```python
from build123d import *

# Parameters (mm, degrees)
SKETCH1_W           = 110
SKETCH1_H           = 150
BOSS_EXTRUDE1_DEPTH = 10
SKETCH2_W           = 9.95
SKETCH2_H           = 11
BOSS_EXTRUDE2_DEPTH = 7
SKETCH3_W           = 19.95
SKETCH3_H           = 11
SKETCH3_W_2         = 20
BOSS_EXTRUDE3_DEPTH = 6.95
SKETCH6_R           = 1.425
CUT_EXTRUDE1_DEPTH  = 10
SKETCH7_W           = 110
SKETCH7_H           = 1
BOSS_EXTRUDE4_DEPTH = 2


with BuildPart() as part:
    # Sketch1 → Boss-Extrude1 (new body)
    with BuildSketch(Plane.XY):
        with Locations((-38.267930395, -69.615981522)):
            Rectangle(SKETCH1_W, SKETCH1_H)
    extrude(amount=BOSS_EXTRUDE1_DEPTH)

    # Sketch2 → Boss-Extrude2 (add)
    with BuildSketch(Plane.XY.offset(10)):
        with Locations((-63.252930395, -0.115981522)):
            Rectangle(SKETCH2_W, SKETCH2_H)
        with Locations((-13.302930395, -0.115981522)):
            Rectangle(SKETCH2_W, SKETCH2_H)
    boss_extrude2 = extrude(amount=BOSS_EXTRUDE2_DEPTH)

    # Sketch3 → Boss-Extrude3 (add)
    with BuildSketch(Plane.XY.offset(17)):
        with Locations((-63.252930395, -0.115981522)):
            Rectangle(SKETCH3_W, SKETCH3_H)
        with Locations((-13.307930395, -0.115981522)):
            Rectangle(SKETCH3_W_2, SKETCH3_H)
    boss_extrude3 = extrude(amount=BOSS_EXTRUDE3_DEPTH)

    # Sketch6 → Cut-Extrude1 (cut)
    with BuildSketch(Plane.XY.offset(10)):
        with Locations((-85.267930395, -20.615981522)):
            Circle(SKETCH6_R)
        with Locations((8.732069605, -20.615981522)):
            Circle(SKETCH6_R)
    cut_extrude1 = extrude(amount=-CUT_EXTRUDE1_DEPTH, mode=Mode.SUBTRACT)

    # Sketch7 → Boss-Extrude4 (add)
    with BuildSketch(Plane.XY.offset(10)):
        with Locations((-38.267930395, -18.115981522)):
            Rectangle(SKETCH7_W, SKETCH7_H)
    extrude(amount=BOSS_EXTRUDE4_DEPTH)

    # Mirror1: Boss-Extrude2, Boss-Extrude3, Cut-Extrude1 across plane
    add(boss_extrude2.mirror(Plane(origin=(16.732069605, -17.615981522, 12), x_dir=(0, 0, 1), z_dir=(0, -1, 0))))
    add(boss_extrude3.mirror(Plane(origin=(16.732069605, -17.615981522, 12), x_dir=(0, 0, 1), z_dir=(0, -1, 0))))
    add(cut_extrude1.mirror(Plane(origin=(16.732069605, -17.615981522, 12), x_dir=(0, 0, 1), z_dir=(0, -1, 0))), mode=Mode.SUBTRACT)


solid = part.part
```
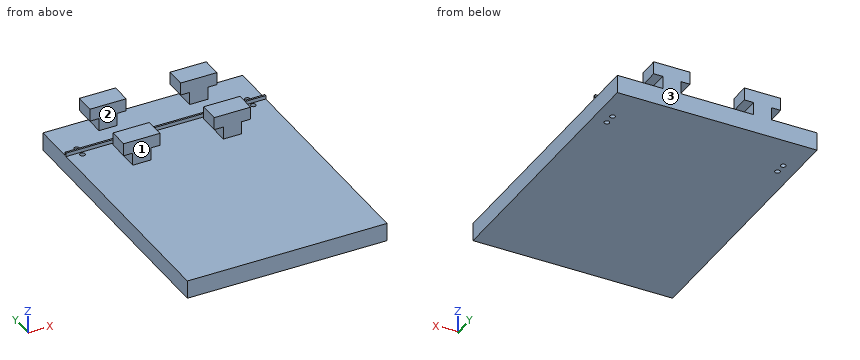
Input: part model. Units: mm. Frame: model coordinates. Face numbers are marked on the shaded views. A direction names the side the tool comes from. Give positions to 0.01 mm unless a question says otherwise; leave off trailing zeros. Order: outer loops, then holes, each group sorted by start corner. A loop starts at its lowest first (then second) coordinate and runs counter-clockwise, first axis right, second up. Notation, with made-up numbers: (-12, -30.75) - (5, -30.75) arc R28 ccw to (5, -4.75) - close; hole circle Ø4 at (59.5, 35.5). An arc over 180 degrees is marked (long way). Use a Markdown table: item, result.
(1) Section query C-C (y = -11). Output: boundary loops of the cut face in (x, z), then the cut area to 3 significant figures.
Computed values:
| item | result |
|---|---|
| outline | (-93.27, 0) - (16.73, 0) - (16.73, 10) - (-93.27, 10) - close |
| area | 1,100 mm2 |
(2) Section query B-B (x = -14.5). Output: boundary loops of the cut face in (y, z).
Computed values:
| item | result |
|---|---|
| outline | (-144.62, 0) - (5.38, 0) - (5.38, 23.95) - (-5.62, 23.95) - (-5.62, 10) - (-17.62, 10) - (-17.62, 12) - (-18.62, 12) - (-18.62, 10) - (-29.62, 10) - (-29.62, 23.95) - (-40.62, 23.95) - (-40.62, 10) - (-144.62, 10) - close |
(3) Section query D-D (z = 22.25). Output: boundary loops of the cut face in (x, y), then the cut area to 3 significant figures.
Computed values:
| item | result |
|---|---|
| outline | (-73.23, -40.62) - (-53.28, -40.62) - (-53.28, -29.62) - (-73.23, -29.62) - close; (-73.23, -5.62) - (-53.28, -5.62) - (-53.28, 5.38) - (-73.23, 5.38) - close; (-23.31, -40.62) - (-3.31, -40.62) - (-3.31, -29.62) - (-23.31, -29.62) - close; (-23.31, -5.62) - (-3.31, -5.62) - (-3.31, 5.38) - (-23.31, 5.38) - close |
| area | 879 mm2 |
(4) Access query for the marked faces 1, 2 and 3. Directions: +Z, -Z, +X, -X, +Y, -Y. A direction counts if a zero-diameter tool reaches every point of the face in a straight line with its end or side. Return the directions, or none.
Computed values:
| item | result |
|---|---|
| face 1 | +Z, +X, -X, -Y |
| face 2 | +Z, +X, -X |
| face 3 | +Z, -Z, +X, -X, +Y |
(5) Line query: line 1 (X direction, y = -31, z = 14.5); line 2 (Y direction, x = -72, z = 20.5); line 3 (Z direction, x = 1, y = -109.5). Output: solid intervals per line, ascending. Write a range as from..to.
Computed values:
| item | result |
|---|---|
| line 1 | x = -68.23..-58.28, -18.28..-8.33 |
| line 2 | y = -40.62..-29.62, -5.62..5.38 |
| line 3 | z = 0..10 |
(6) Pin query (flat end, axial travel): pin 1 (2 mm diameter, centred on y = -37, z = 19, fed in from -X); pin 2 (5.5 mm diameter, centred on y = -38, z = 13, fed in from +X); pin 3 (2 mm diameter, centred on y = -2, z = 12, fed in from -X); pin 4 (1.7 mm diameter, centred on x = 8.73, y = -20.62, fed in from -Z). Return the tip coordinate at first contact, or that it passes through.
Computed values:
| item | result |
|---|---|
| pin 1 | stops at x = -73.23 |
| pin 2 | stops at x = -8.33 |
| pin 3 | stops at x = -68.23 |
| pin 4 | passes through |
(7) Section query A-A (z = 13.75). Output: boundary loops of the cut face in (x, y), then the cut area to 3 significant figures.
Computed values:
| item | result |
|---|---|
| outline | (-68.23, -40.62) - (-58.28, -40.62) - (-58.28, -29.62) - (-68.23, -29.62) - close; (-68.23, -5.62) - (-58.28, -5.62) - (-58.28, 5.38) - (-68.23, 5.38) - close; (-18.28, -40.62) - (-8.33, -40.62) - (-8.33, -29.62) - (-18.28, -29.62) - close; (-18.28, -5.62) - (-8.33, -5.62) - (-8.33, 5.38) - (-18.28, 5.38) - close |
| area | 438 mm2 |
